Drawing for the job (mm, zero at the part's lowest x, y, z). A direction names the side the tool comes from. Coordinates: 2 decimals unless noted, no trailing zeros. Loops run counter-clockwise (first coordinate to the right, second up) from the corner with the lowest first, then second, coordinate; pieces in that order, holes last.
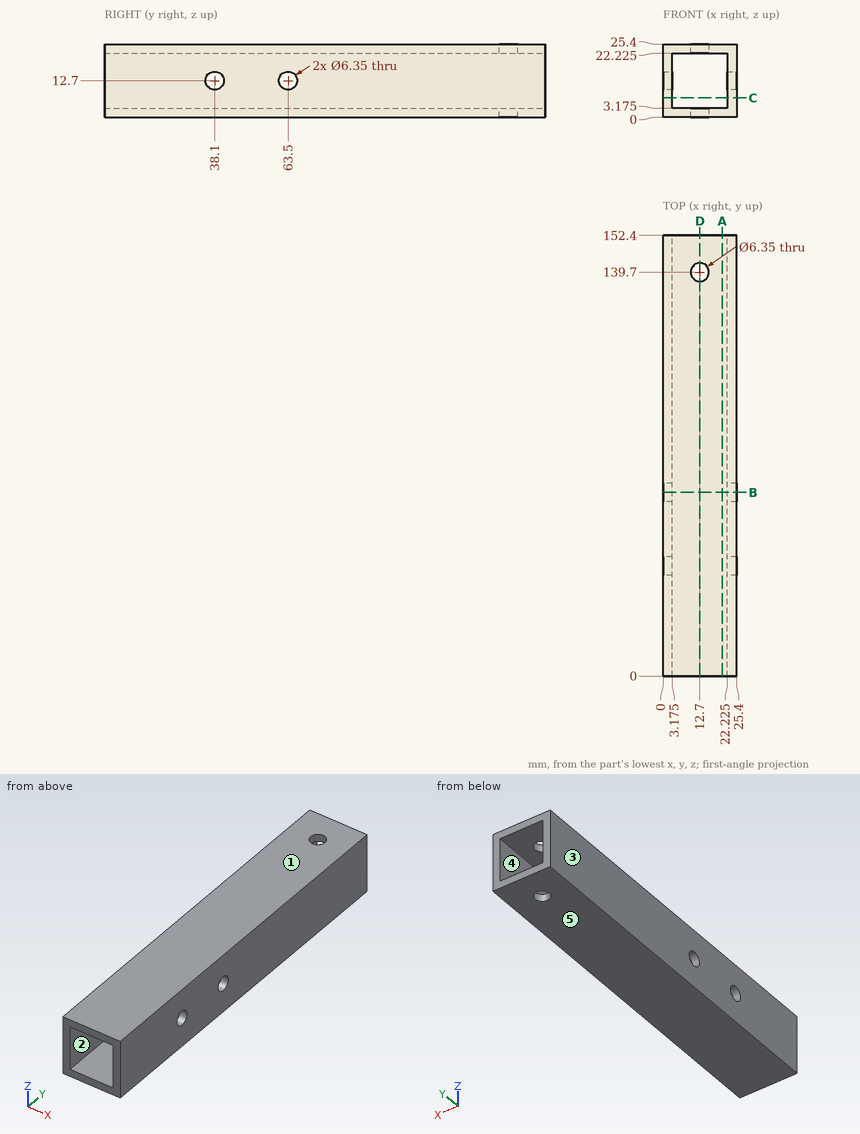
Q1. Saw through at D-D (x = 12.7). List the corners of the cut face in (y, z) (3 decimals), plus the area to 3 significant figures.
Q2. Saw through at A-A (x = 20.5). List the corners of the cut face in (y, z) (3 decimals).
Q3. Tool access for the marked faces 1 and 2: list every direction of +Z, -Z, +X, -X, +Y, -Y with a clear straight run to the whole face (end or side of a thin tool).
Q4. Mould opens along X. For the marked faces 3, 4 and 5 say: released by +X, released by -X, zero draft, split by the parting line, or undercut.
Q5. Saw through at B-B (y = 63.5). List the corners of the cut face in (x, z) (3 decimals).
Q6. Saw through at C-C (z = 6.75). List the corners of the cut face in (x, y) (3 decimals), plus the area to 3 significant figures.
Q7. Drop a flat-ended pin along its axis: P1, Ø12, axis at x = 17, z = 6, coming from the -Y side. Give the stop position or say it passes through.
Q8. Probe line 1 (Y direction, x = 2.1, z = 12.7) (3 decimals); line 2 (X direction, y = 134, z = 8) (3 decimals). List the from-to ranges inside material, lowest first.
Checked values:
1. outline: (0, 0) - (136.525, 0) - (136.525, 3.175) - (0, 3.175) - close; (0, 22.225) - (136.525, 22.225) - (136.525, 25.4) - (0, 25.4) - close; (142.875, 0) - (152.4, 0) - (152.4, 3.175) - (142.875, 3.175) - close; (142.875, 22.225) - (152.4, 22.225) - (152.4, 25.4) - (142.875, 25.4) - close
1. area: 927 mm2
2. outline: (0, 0) - (152.4, 0) - (152.4, 3.175) - (0, 3.175) - close; (0, 22.225) - (152.4, 22.225) - (152.4, 25.4) - (0, 25.4) - close
3. face 1: +Z, +X, -X, +Y, -Y
3. face 2: +Y, -Y
4. face 3: released by -X
4. face 4: undercut
4. face 5: zero draft
5. outline: (0, 0) - (25.4, 0) - (25.4, 9.525) - (22.225, 9.525) - (22.225, 3.175) - (3.175, 3.175) - (3.175, 9.525) - (0, 9.525) - close; (0, 15.875) - (3.175, 15.875) - (3.175, 22.225) - (22.225, 22.225) - (22.225, 15.875) - (25.4, 15.875) - (25.4, 25.4) - (0, 25.4) - close
6. outline: (0, 0) - (3.175, 0) - (3.175, 152.4) - (0, 152.4) - close; (22.225, 0) - (25.4, 0) - (25.4, 152.4) - (22.225, 152.4) - close
6. area: 968 mm2
7. P1: stops at y = 0
8. line 1: y = 0 to 34.925, 41.275 to 60.325, 66.675 to 152.4
8. line 2: x = 0 to 3.175, 22.225 to 25.4
